Could you check a few things on this model? Use its own coordinates, in mm. Face numbers are marked on the shaded views. A direction names the side the tool comes from. Coordinates: 2 decimals unless noted, no trailing zeros. Order: outer loops, then holes, each group sorted by start corner. A loop starts at its lowest first (then second) coordinate and runs counter-clockwise, first axis right, second up. Notation, with made-up numbers: (30.25, 85) -> (49.25, 85) arc R22 cw to (49.25, 104) -> close; hole circle Ø10 at (20.25, 36.25). An arc over 180 degrees is marked (long way). Return JSON: item names as keys, results as strings. Group by question number.
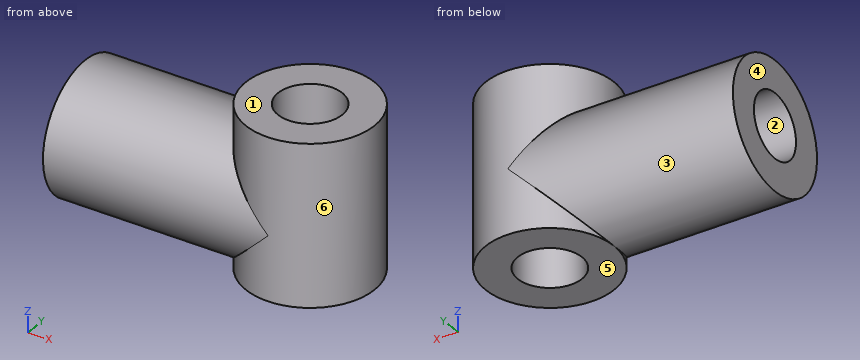
from build123d import *

# Parameters (mm, degrees)
SKETCH1_R           = 6
SKETCH1_R_2         = 3
BOSS_EXTRUDE1_DEPTH = 15
SKETCH2_R           = 6
SKETCH2_R_2         = 3
BOSS_EXTRUDE2_DEPTH = 21
SKETCH3_R           = 3
CUT_EXTRUDE1_DEPTH  = 16.0000001


with BuildPart() as part:
    # Sketch1 → Boss-Extrude1 (new body)
    with BuildSketch(Plane.XY):
        Circle(SKETCH1_R)
        Circle(SKETCH1_R_2, mode=Mode.SUBTRACT)
    extrude(amount=BOSS_EXTRUDE1_DEPTH)

    # Sketch2 → Boss-Extrude2 (add)
    with BuildSketch(Plane(origin=(0, 0, 0), x_dir=(0, 0, -1), z_dir=(1, 0, 0))):
        with Locations((-6, 0)):
            Circle(SKETCH2_R)
        with Locations((-6, 0)):
            Circle(SKETCH2_R_2, mode=Mode.SUBTRACT)
    extrude(amount=-BOSS_EXTRUDE2_DEPTH)

    # Sketch3 → Cut-Extrude1 (cut, through all)
    with BuildSketch(Plane(origin=(0, 0, 0), x_dir=(-1, 0, 0), z_dir=(0, 0, -1))):
        Circle(SKETCH3_R)
    extrude(amount=-CUT_EXTRUDE1_DEPTH, mode=Mode.SUBTRACT)


solid = part.part
Q1. I need wall thicknesses on line 1 along Y through (x, z) = (-15, 6); line 2 along Z through (x, y) = (-17.25, 0); line 3 along X through (y, z) = (-1.5, 1.25). Which ranges of each line are inside material? Lowest first, please. Write a range as from..to.
Q2. On a 3-axis mill with a long thin cutter (end or side, diameter ignored), from which of +Z, -Z, +X, -X, +Y, -Y can I reach the whole of each face in a straight line? I mean the marked faces 5 and 6. Say none if no direction works.
Q3. I want a section at D-D on y = 5.25. Please give me the cut outline in (x, z), and give its area (3 significant figures).
Q4. I'm going to push flat-ended pins straight in: pin 1 Ø1.5 at (x, z) = (-9, 5) entering from -Y; pin 2 Ø6 at (x, z) = (-13, 5) entering from +Y; pin 3 Ø2 at (y, z) = (3, 9) entering from +X; pin 4 Ø6 at (x, z) = (-11.5, 11) entering from -Y. Where does each tip first touch, or does it pass through?
Q5. I want a section at C-C on x = -15.25. Please give me the cut outline in (y, z).
Q6. I want a section at B-B on z = 6. Please give me the cut outline in (x, y).
Q7. We'd pull the mould along Z, two halves only. Please class the marked faces 1, 2, 3 and 4: pulls with the +Z half, pulls with the -Z half, needs draft (parallel to the pull), parting line crosses it, or undercut.
Response values:
{
 "1": {"line 1": "y = -6..-3, 3..6", "line 2": "z = 0..3, 9..12", "line 3": "x = -21..-2.6, 2.6..5.81"},
 "2": {"face 5": "-Z, +X, -X, +Y, -Y", "face 6": "none"},
 "3": {"outline": "(-21, 3.1) -> (-2.9, 3.1) -> (-2.9, 0) -> (2.9, 0) -> (2.9, 15) -> (-2.9, 15) -> (-2.9, 8.9) -> (-21, 8.9) -> close", "area": "192 mm²"},
 "4": {"pin 1": "stops at y = -5.99", "pin 2": "stops at y = 6", "pin 3": "stops at x = 5.66", "pin 4": "stops at y = -5.66"},
 "5": {"outline": "circle Ø12 at (0, 6); hole circle Ø6 at (0, 6)"},
 "6": {"outline": "(-21, -6) -> (0, -6) arc R6 ccw to (0, 6) -> (-21, 6) -> (-21, 3) -> (-5.2, 3) arc R6 ccw to (-5.2, -3) -> (-21, -3) -> close; hole circle Ø6 at (0, 0)"},
 "7": {"face 1": "pulls with the +Z half", "face 2": "undercut", "face 3": "parting line crosses it", "face 4": "needs draft"}
}
